Geometry: final body of the model. Coordinates: model frame, mm. A direction names the side the tool comes from. Round coordinates to 2 decimals unless told otherwise and drop trailing zeros. Write each loop counter-clockwise with the first axis right and the second up, starting at its lowest first coordinate (ties: lowest second). Pieces come first, ordered by that corner, then holes.
from build123d import *

# Parameters (mm, degrees)
F0_R     = 4
F0_R_2   = 22.606
F1_DEPTH = 12


with BuildPart() as f1:
    # F0 (on Front) → F1 (new body)
    with BuildSketch(Plane.XZ):
        with BuildLine():
            ThreePointArc((17.802502, 144.956856), (11.512632, 149.678862), (7.529827, 156.460976))
            Line((7.529827, 156.460976), (2.835124, 170.030854))
            ThreePointArc((2.835124, 170.030854), (0, 172.05), (-2.835124, 170.030854))
            Line((-2.835124, 170.030854), (-7.529827, 156.460976))
            ThreePointArc((-7.529827, 156.460976), (-11.512632, 149.678862), (-17.802502, 144.956856))
            ThreePointArc((-17.802502, 144.956856), (-30.241911, 141.830071), (-43.068077, 141.901717))
            ThreePointArc((-43.068077, 141.901717), (-48.22329, 144.439154), (-52.558881, 148.209759))
            Line((-52.558881, 148.209759), (-63.367118, 160.390291))
            ThreePointArc((-63.367118, 160.390291), (-66.759125, 161.170784), (-68.605744, 158.220382))
            Line((-68.605744, 158.220382), (-67.53653, 143.678524))
            ThreePointArc((-67.53653, 143.678524), (-68.731889, 135.702982), (-73.239492, 129.015707))
            ThreePointArc((-73.239492, 129.015707), (-81.548929, 122.076108), (-91.140166, 117.054859))
            ThreePointArc((-91.140166, 117.054859), (-99.243222, 115.675861), (-107.216606, 117.672431))
            Line((-107.216606, 117.672431), (-119.808645, 123.791189))
            ThreePointArc((-119.808645, 123.791189), (-123.3221, 123.180437), (-123.769366, 119.642452))
            Line((-123.769366, 119.642452), (-117.840644, 107.121025))
            ThreePointArc((-117.840644, 107.121025), (-115.861515, 99.254778), (-117.195431, 91.253812))
            ThreePointArc((-117.195431, 91.253812), (-122.21668, 81.662575), (-129.156279, 73.353138))
            ThreePointArc((-129.156279, 73.353138), (-136.114807, 68.978205), (-144.245307, 67.771513))
            Line((-144.245307, 67.771513), (-158.220382, 68.605744))
            ThreePointArc((-158.220382, 68.605744), (-161.170784, 66.759125), (-160.390291, 63.367118))
            Line((-160.390291, 63.367118), (-149.918532, 54.075138))
            ThreePointArc((-149.918532, 54.075138), (-145.022659, 47.472746), (-143.195782, 39.458779))
            ThreePointArc((-143.195782, 39.458779), (-144.164403, 28.676083), (-147.395873, 18.343495))
            ThreePointArc((-147.395873, 18.343495), (-152.1505, 11.638671), (-159.200322, 7.412425))
            Line((-159.200322, 7.412425), (-172.430854, 2.835124))
            ThreePointArc((-172.430854, 2.835124), (-174.45, 0), (-172.430854, -2.835124))
            Line((-172.430854, -2.835124), (-159.200322, -7.412425))
            ThreePointArc((-159.200322, -7.412425), (-152.1505, -11.638671), (-147.395873, -18.343495))
            ThreePointArc((-147.395873, -18.343495), (-144.164403, -28.676083), (-143.195782, -39.458779))
            ThreePointArc((-143.195782, -39.458779), (-145.022659, -47.472746), (-149.918532, -54.075138))
            Line((-149.918532, -54.075138), (-160.390291, -63.367118))
            ThreePointArc((-160.390291, -63.367118), (-161.170784, -66.759125), (-158.220382, -68.605744))
            Line((-158.220382, -68.605744), (-144.245307, -67.771513))
            ThreePointArc((-144.245307, -67.771513), (-136.114807, -68.978205), (-129.156279, -73.353138))
            ThreePointArc((-129.156279, -73.353138), (-122.21668, -81.662575), (-117.195431, -91.253812))
            ThreePointArc((-117.195431, -91.253812), (-115.816433, -99.356868), (-117.813003, -107.330252))
            Line((-117.813003, -107.330252), (-123.931761, -119.922291))
            ThreePointArc((-123.931761, -119.922291), (-123.354778, -123.354778), (-119.922291, -123.931761))
            Line((-119.922291, -123.931761), (-107.330252, -117.813003))
            ThreePointArc((-107.330252, -117.813003), (-99.356868, -115.816433), (-91.253812, -117.195431))
            ThreePointArc((-91.253812, -117.195431), (-81.662575, -122.21668), (-73.353138, -129.156279))
            ThreePointArc((-73.353138, -129.156279), (-68.978205, -136.114807), (-67.771513, -144.245307))
            Line((-67.771513, -144.245307), (-68.605744, -158.220382))
            ThreePointArc((-68.605744, -158.220382), (-66.759125, -161.170784), (-63.367118, -160.390291))
            Line((-63.367118, -160.390291), (-54.075138, -149.918532))
            ThreePointArc((-54.075138, -149.918532), (-47.615399, -144.248208), (-39.458779, -141.537052))
            ThreePointArc((-39.458779, -141.537052), (-28.676083, -142.505673), (-18.343495, -145.737143))
            ThreePointArc((-18.343495, -145.737143), (-11.638671, -150.49177), (-7.412425, -157.541592))
            Line((-7.412425, -157.541592), (-2.835124, -170.772123))
            ThreePointArc((-2.835124, -170.772123), (0, -172.79127), (2.835124, -170.772123))
            Line((2.835124, -170.772123), (6.228962, -157.864794))
            ThreePointArc((6.228962, -157.864794), (10.92106, -150.437277), (18.343495, -145.737143))
            ThreePointArc((18.343495, -145.737143), (28.766653, -143.349083), (39.458779, -143.195782))
            ThreePointArc((39.458779, -143.195782), (47.472746, -145.022659), (54.075138, -149.918532))
            Line((54.075138, -149.918532), (63.367118, -160.390291))
            ThreePointArc((63.367118, -160.390291), (66.759125, -161.170784), (68.605744, -158.220382))
            Line((68.605744, -158.220382), (67.771513, -144.245307))
            ThreePointArc((67.771513, -144.245307), (68.978205, -136.114807), (73.353138, -129.156279))
            ThreePointArc((73.353138, -129.156279), (81.662575, -122.21668), (91.253812, -117.195431))
            ThreePointArc((91.253812, -117.195431), (99.356868, -115.816433), (107.330252, -117.813003))
            Line((107.330252, -117.813003), (119.922291, -123.931761))
            ThreePointArc((119.922291, -123.931761), (123.354778, -123.354778), (123.931761, -119.922291))
            Line((123.931761, -119.922291), (117.813003, -107.330252))
            ThreePointArc((117.813003, -107.330252), (115.816433, -99.356868), (117.195431, -91.253812))
            ThreePointArc((117.195431, -91.253812), (122.21668, -81.662575), (129.156279, -73.353138))
            ThreePointArc((129.156279, -73.353138), (136.114807, -68.978205), (144.245307, -67.771513))
            Line((144.245307, -67.771513), (158.220382, -68.605744))
            ThreePointArc((158.220382, -68.605744), (161.170784, -66.759125), (160.390291, -63.367118))
            Line((160.390291, -63.367118), (149.918532, -54.075138))
            ThreePointArc((149.918532, -54.075138), (145.022659, -47.472746), (143.195782, -39.458779))
            ThreePointArc((143.195782, -39.458779), (144.164403, -28.676083), (147.395873, -18.343495))
            ThreePointArc((147.395873, -18.343495), (152.1505, -11.638671), (159.200322, -7.412425))
            Line((159.200322, -7.412425), (172.430854, -2.835124))
            ThreePointArc((172.430854, -2.835124), (174.45, 0), (172.430854, 2.835124))
            Line((172.430854, 2.835124), (159.200322, 7.412425))
            ThreePointArc((159.200322, 7.412425), (152.1505, 11.638671), (147.395873, 18.343495))
            ThreePointArc((147.395873, 18.343495), (144.164403, 28.676083), (143.195782, 39.458779))
            ThreePointArc((143.195782, 39.458779), (145.022659, 47.472746), (149.918532, 54.075138))
            Line((149.918532, 54.075138), (160.390291, 63.367118))
            ThreePointArc((160.390291, 63.367118), (161.170784, 66.759125), (158.220382, 68.605744))
            Line((158.220382, 68.605744), (144.245307, 67.771513))
            ThreePointArc((144.245307, 67.771513), (136.114807, 68.978205), (129.156279, 73.353138))
            ThreePointArc((129.156279, 73.353138), (122.222235, 81.705182), (117.22101, 91.339774))
            ThreePointArc((117.22101, 91.339774), (115.842012, 99.442829), (117.838582, 107.416213))
            Line((117.838582, 107.416213), (123.95734, 120.008252))
            ThreePointArc((123.95734, 120.008252), (123.380357, 123.44074), (119.94787, 124.017723))
            Line((119.94787, 124.017723), (107.35583, 117.898965))
            ThreePointArc((107.35583, 117.898965), (99.382446, 115.902395), (91.279391, 117.281393))
            ThreePointArc((91.279391, 117.281393), (82.47428, 120.828447), (74.484519, 125.95439))
            ThreePointArc((74.484519, 125.95439), (70.109586, 132.912918), (68.902895, 141.043418))
            Line((68.902895, 141.043418), (69.737125, 155.018493))
            ThreePointArc((69.737125, 155.018493), (67.890506, 157.968896), (64.498499, 157.188402))
            Line((64.498499, 157.188402), (55.206519, 146.716643))
            ThreePointArc((55.206519, 146.716643), (48.58216, 141.810683), (40.541822, 139.993122))
            ThreePointArc((40.541822, 139.993122), (28.884055, 141.155145), (17.802502, 144.956856))
        make_face()
        with Locations((-30.310889, -17.5)):
            Circle(F0_R, mode=Mode.SUBTRACT)
        with Locations((0, -100)):
            Circle(F0_R, mode=Mode.SUBTRACT)
        with Locations((30.310889, -17.5)):
            Circle(F0_R, mode=Mode.SUBTRACT)
        with Locations((-86.60254, 50)):
            Circle(F0_R, mode=Mode.SUBTRACT)
        Circle(F0_R_2, mode=Mode.SUBTRACT)
        with Locations((0, 35)):
            Circle(F0_R, mode=Mode.SUBTRACT)
        with Locations((86.60254, 50)):
            Circle(F0_R, mode=Mode.SUBTRACT)
    extrude(amount=F1_DEPTH)


solid = f1.part
1) Section C-C on z = -100. Output: boundary loops of the cut face in (x, y), plus the area to 3 significant figures.
2) Section D-D on y = -6. State how many separate pieces and enclosed holes the cut face has, plus the area to 3 significant figures.
3) First-contact query: P1, Ø13, axis at x = 0, z = 35, coming from the +Y side; P2, Ø1, axis at y = -8.5, z = 56.5, coming from the +X side; P3, Ø3, axis at y = -6.5, z = 40.5, coming from the -X side; P4, Ø6, axis at y = -8, z = 128, coming from the +X side. Flat tips, straight axial feed; report the tip coordinate or a pass-through.
4) Reachability of faces 5 (the flat face through (-5.156, -5.916, -164.064)), 6 (the flat face through (59.92, -5.92, 152.03)), 7 (the flat face through (-120.83, -5.92, -113.54)), 8 (the flat face through (155.081, -5.916, 58.656)) from +Z, -Z, +X, -X, +Y, -Y: full face, straight path, thin tool, end or side. Return the list, or none.
5) Draft query along Z for faces 1 (the cylindrical face through (-152.236, -5.916, -11.56)), 2 (the cylindrical face through (-47.72, -5.92, -144.31)), 3 (the cylindrical face through (-99.13, -5.92, 115.67)), 4 (the cylindrical face through (-144.2, -5.9, -28.5)). Return one class per face: pulls with the +Z half, pulls with the -Z half, needs draft (parallel to the pull), parting line crosses it, or undercut.
6) Section B-B on z = 50. Output: boundary loops of the cut face in (x, y).
7) Section A-A on x = -12.5. Output: boundary loops of the cut face in (y, z), plus the area to 3 significant figures.
8) Line query: probe 1 along Z at (x, y) = (0, -7.75); probe 2 along X at (y, z) = (-0.25, 53); probe 3 along X at (y, z) = (-2.75, -123.5). Output: solid intervals per line, ascending.
Filled in:
1. outline: (-115.85, -12) - (-4, -12) - (-4, 0) - (-115.85, 0) - close; (4, -12) - (115.85, -12) - (115.85, 0) - (4, 0) - close
1. area: 2,680 mm2
2. separate pieces: 1
2. enclosed holes: 7
2. area: 72,700 mm2
3. P1: stops at y = 0
3. P2: stops at x = 153.21
3. P3: stops at x = -143.4
3. P4: stops at x = 75.74
4. face 5: -Z, +Y, -Y
4. face 6: +Z, +Y, -Y
4. face 7: -X, +Y, -Y
4. face 8: +X, +Y, -Y
5. face 1: undercut
5. face 2: pulls with the -Z half
5. face 3: pulls with the +Z half
5. face 4: undercut
6. outline: (-146.41, -12) - (-90.6, -12) - (-90.6, 0) - (-146.41, 0) - close; (-82.6, -12) - (82.6, -12) - (82.6, 0) - (-82.6, 0) - close; (90.6, -12) - (146.41, -12) - (146.41, 0) - (90.6, 0) - close
7. outline: (-12, -149.62) - (0, -149.62) - (0, -18.84) - (-12, -18.84) - close; (-12, 18.84) - (0, 18.84) - (0, 148.65) - (-12, 148.65) - close
7. area: 3,130 mm2
8. probe 1: z = -172.79 to -104, -96 to -22.61, 22.61 to 31, 39 to 172.05
8. probe 2: x = -148.8 to -89.25, -83.96 to 83.96, 89.25 to 148.8
8. probe 3: x = -123.2 to -119.03, -79.83 to 79.83, 119.03 to 123.2
